Input: dimensioned drawing with shaded views. Units: mm. Origin: part minimum x, y, z. A direction names the side the tool comes from. Round coordinates to 2 decimals unless told otherwise and drop trailing zeros. Order: outer loops, then holes, each group sorted by start corner. A loop starts at its lowest first (then second) coordinate and runs counter-clockwise, first axis right, second up. Notation, with made-up numbers: M 82.25,25 L 118.25,25 A36 cw 118.25,64 Z; hole C -21,68 d3. An arc over 180 degrees is marked long. Put each result on its own line as item: value. Start each with the question number.
1) Section A-A, the plane y = 28.5. Return loops of the section in (x, z).
2) Section B-B, the plane x = 5. Return loops of the section in (y, z).
3) Material intervals for probe 1 along Y at (x, z) = (5, 3.25); probe 2 along Y at (x, z) = (19, 2.75), sorted ascending. Write a range as [from, to].
4) First-contact query: P1, Ø3, axis at y = 38, z = 1, coming from the +X side; P2, Ø3.5, axis at x = 5, y = 5, coming from the -Z side; P3, Ø3, axis at y = 47, z = 3.5, coming from the +X side; P4, Ø3, axis at x = 24, z = 1.5, coming from the -Y side. Flat tips, straight axial feed; report the tip coordinate or a pass-through.
5) Draft query along X for the marked faces 4, 5 and 6. Return one class per face: pulls with the +X half, pulls with the -X half, needs draft (parallel to the pull), parting line crosses it, or undercut.
6) Access query for the marked faces 1, 2 and 3. Directions: +Z, -Z, +X, -X, +Y, -Y. A direction counts if a zero-diameter tool reaches every point of the face in a straight line with its end or side. Return the directions, or none.
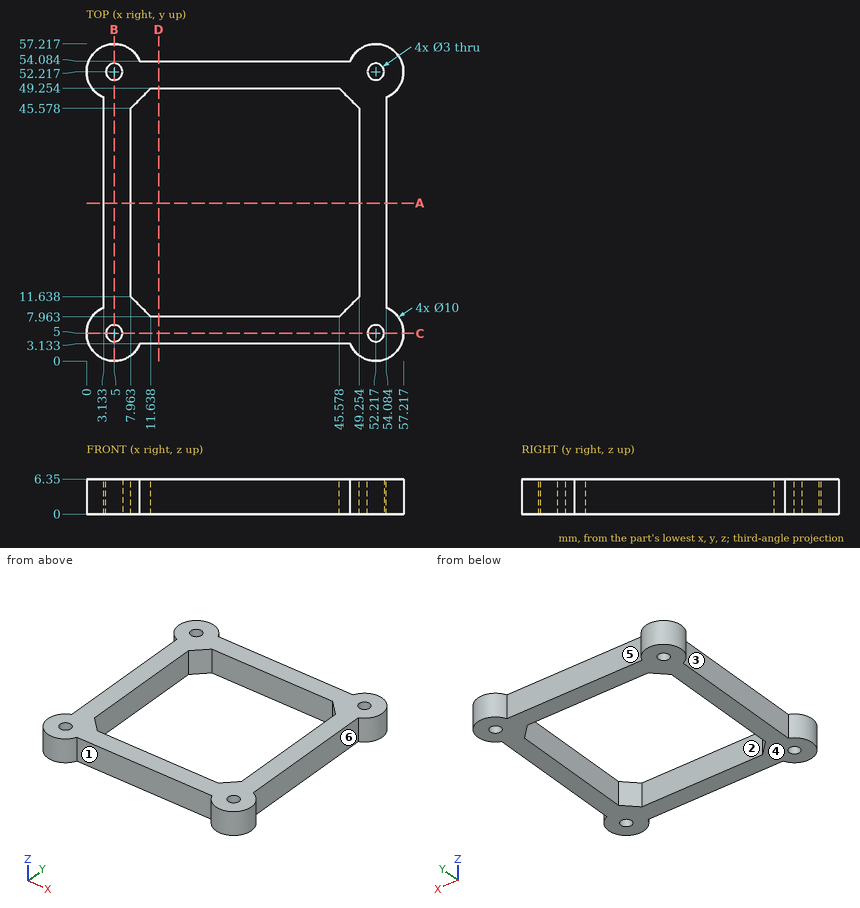
Result sheet:
1. outline: M 3.13,0 L 7.96,0 L 7.96,6.35 L 3.13,6.35 Z; M 49.25,0 L 54.08,0 L 54.08,6.35 L 49.25,6.35 Z
2. outline: M 0,0 L 3.5,0 L 3.5,6.35 L 0,6.35 Z; M 6.5,0 L 50.72,0 L 50.72,6.35 L 6.5,6.35 Z; M 53.72,0 L 57.22,0 L 57.22,6.35 L 53.72,6.35 Z
3. probe 1: y = [0, 3.5], [6.5, 50.72], [53.72, 57.22]
3. probe 2: y = [3.13, 7.96], [49.25, 54.08]
4. P1: stops at x = 54.08
4. P2: stops at z = 0
4. P3: stops at x = 55.56
4. P4: stops at y = 3.13
5. face 4: needs draft
5. face 5: undercut
5. face 6: pulls with the +X half
6. face 1: +Z, -Z, -Y
6. face 2: +Z, -Z
6. face 3: +Z, -Z, -X
